Can you work these out from the model? Positions are in its coordinate system, mm. A direction names the side the tool comes from. Round coordinates to 2 decimals unless told otherwise and drop trailing zeros. Write each loop counter-clockwise with the first axis right and the second up, starting at its lowest first coordinate (ties: lowest second). Pieces come first, ordered by that corner, then holes. Notation, with made-up numbers: (-19.75, 58.25) - (-10.75, 58.25) arc R7 ccw to (-10.75, 70.25) - close; hole circle Ø7 at (56, 66.5). An arc over 180 degrees is marked (long way). One line per item, written item: value. Start each with the question number.
(1) On a 3-axis mill with a long thin cutter (end or side, diameter ignored), from which of +Z, -Z, +X, -X, +Y, -Y can I reach the whole of each face in a straight line? I mean faces 4 (the face through (6, 101, 12.7)), 5 (the face through (-10, 99, 15)). Say none if no direction works.
(2) I want a section at B-B on z = 0. List the corners of the cut face in (x, y) for me.
(3) Thinking about a two-plate mould opening in Z: for faces 1 (the face through (-7.83, 101.4, -6.38)), 2 (the face through (9, 99, -15)), 3 (the face through (15, 99, 10)), which applies, +Z half, -Z half, draft (parallel to the pull), parting line (faces both ways), or undercut?
(4) I'm going to push flat-ended pins straight in: pin 1 Ø4.5 at (y, z) = (75, 0.5) entering from +X; pin 2 Ø4.5 at (x, y) = (-0.5, 116) entering from -Z. Where does each tip first touch, or does it pass through?
(5) I want a section at A-A on x = 0. List the corners of the cut face in (y, z) for me, plus the area to 3 significant figures.
(6) If I drill on L1, parallel to X at y = 55, z = -11.75; L2, parallel to Z at x = 4.5, y = 11.5, over which ranges is the centre line in solid material (lowest first)? Write a range as from..to.
from build123d import *

# Parameters (mm, degrees)
CROQUIS1_W              = 30
CROQUIS1_H              = 30
SALIENTE_EXTRUIR1_DEPTH = 200
CROQUIS3_R              = 3.5
CORTAR_EXTRUIR2_DEPTH   = 202.121853611


with BuildPart() as part:
    # Croquis1 → Saliente-Extruir1 (new body)
    with BuildSketch(Plane(origin=(0, 0, 0), x_dir=(1, 0, 0), z_dir=(0, 1, 0))):
        Rectangle(CROQUIS1_W, CROQUIS1_H)
    extrude(amount=SALIENTE_EXTRUIR1_DEPTH)

    # Croquis3 → Cortar-Extruir2 (cut, through all)
    with BuildSketch(Plane(origin=(0, 200, 0), x_dir=(1, 0, 0), z_dir=(0, 1, 0))):
        with Locations(Location((0, 0, 0), (0, 0, 270))):
            Circle(CROQUIS3_R)
        with BuildLine():
            Line((4, 15), (-4, 15))
            Line((-4, 15), (-4, 13.2))
            ThreePointArc((-4, 13.2), (-4.146446609, 12.846446609), (-4.5, 12.7))
            Line((-4.5, 12.7), (-7.75, 12.7))
            ThreePointArc((-7.75, 12.7), (-8.103553391, 12.553553391), (-8.25, 12.2))
            Line((-8.25, 12.2), (-8.25, 9.907106781))
            ThreePointArc((-8.25, 9.907106781), (-8.211939766, 9.715765065), (-8.103553391, 9.553553391))
            Line((-8.103553391, 9.553553391), (-4.696446609, 6.146446609))
            ThreePointArc((-4.696446609, 6.146446609), (-4.534234935, 6.038060234), (-4.342893219, 6))
            Line((-4.342893219, 6), (4.342893219, 6))
            ThreePointArc((4.342893219, 6), (4.534234935, 6.038060234), (4.696446609, 6.146446609))
            Line((4.696446609, 6.146446609), (8.103553391, 9.553553391))
            ThreePointArc((8.103553391, 9.553553391), (8.211939766, 9.715765065), (8.25, 9.907106781))
            Line((8.25, 9.907106781), (8.25, 12.2))
            ThreePointArc((8.25, 12.2), (8.103553391, 12.553553391), (7.75, 12.7))
            Line((7.75, 12.7), (4.5, 12.7))
            ThreePointArc((4.5, 12.7), (4.146446609, 12.846446609), (4, 13.2))
            Line((4, 13.2), (4, 15))
        make_face()
        with BuildLine():
            Line((6, 4.342893219), (6, -4.342893219))
            ThreePointArc((6, -4.342893219), (6.038060234, -4.534234935), (6.146446609, -4.696446609))
            Line((6.146446609, -4.696446609), (9.553553391, -8.103553391))
            ThreePointArc((9.553553391, -8.103553391), (9.715765065, -8.211939766), (9.907106781, -8.25))
            Line((9.907106781, -8.25), (12.2, -8.25))
            ThreePointArc((12.2, -8.25), (12.553553391, -8.103553391), (12.7, -7.75))
            Line((12.7, -7.75), (12.7, -4.5))
            ThreePointArc((12.7, -4.5), (12.846446609, -4.146446609), (13.2, -4))
            Line((13.2, -4), (15, -4))
            Line((15, -4), (15, 4))
            Line((15, 4), (13.2, 4))
            ThreePointArc((13.2, 4), (12.846446609, 4.146446609), (12.7, 4.5))
            Line((12.7, 4.5), (12.7, 7.75))
            ThreePointArc((12.7, 7.75), (12.553553391, 8.103553391), (12.2, 8.25))
            Line((12.2, 8.25), (9.907106781, 8.25))
            ThreePointArc((9.907106781, 8.25), (9.715765065, 8.211939766), (9.553553391, 8.103553391))
            Line((9.553553391, 8.103553391), (6.146446609, 4.696446609))
            ThreePointArc((6.146446609, 4.696446609), (6.038060234, 4.534234935), (6, 4.342893219))
        make_face()
        with BuildLine():
            Line((4.342893219, -6), (-4.342893219, -6))
            ThreePointArc((-4.342893219, -6), (-4.534234935, -6.038060234), (-4.696446609, -6.146446609))
            Line((-4.696446609, -6.146446609), (-8.103553391, -9.553553391))
            ThreePointArc((-8.103553391, -9.553553391), (-8.211939766, -9.715765065), (-8.25, -9.907106781))
            Line((-8.25, -9.907106781), (-8.25, -12.2))
            ThreePointArc((-8.25, -12.2), (-8.103553391, -12.553553391), (-7.75, -12.7))
            Line((-7.75, -12.7), (-4.5, -12.7))
            ThreePointArc((-4.5, -12.7), (-4.146446609, -12.846446609), (-4, -13.2))
            Line((-4, -13.2), (-4, -15))
            Line((-4, -15), (4, -15))
            Line((4, -15), (4, -13.2))
            ThreePointArc((4, -13.2), (4.146446609, -12.846446609), (4.5, -12.7))
            Line((4.5, -12.7), (7.75, -12.7))
            ThreePointArc((7.75, -12.7), (8.103553391, -12.553553391), (8.25, -12.2))
            Line((8.25, -12.2), (8.25, -9.907106781))
            ThreePointArc((8.25, -9.907106781), (8.211939766, -9.715765065), (8.103553391, -9.553553391))
            Line((8.103553391, -9.553553391), (4.696446609, -6.146446609))
            ThreePointArc((4.696446609, -6.146446609), (4.534234935, -6.038060234), (4.342893219, -6))
        make_face()
        with BuildLine():
            Line((-6, -4.342893219), (-6, 4.342893219))
            ThreePointArc((-6, 4.342893219), (-6.038060234, 4.534234935), (-6.146446609, 4.696446609))
            Line((-6.146446609, 4.696446609), (-9.553553391, 8.103553391))
            ThreePointArc((-9.553553391, 8.103553391), (-9.715765065, 8.211939766), (-9.907106781, 8.25))
            Line((-9.907106781, 8.25), (-12.2, 8.25))
            ThreePointArc((-12.2, 8.25), (-12.553553391, 8.103553391), (-12.7, 7.75))
            Line((-12.7, 7.75), (-12.7, 4.5))
            ThreePointArc((-12.7, 4.5), (-12.846446609, 4.146446609), (-13.2, 4))
            Line((-13.2, 4), (-15, 4))
            Line((-15, 4), (-15, -4))
            Line((-15, -4), (-13.2, -4))
            ThreePointArc((-13.2, -4), (-12.846446609, -4.146446609), (-12.7, -4.5))
            Line((-12.7, -4.5), (-12.7, -7.75))
            ThreePointArc((-12.7, -7.75), (-12.553553391, -8.103553391), (-12.2, -8.25))
            Line((-12.2, -8.25), (-9.907106781, -8.25))
            ThreePointArc((-9.907106781, -8.25), (-9.715765065, -8.211939766), (-9.553553391, -8.103553391))
            Line((-9.553553391, -8.103553391), (-6.146446609, -4.696446609))
            ThreePointArc((-6.146446609, -4.696446609), (-6.038060234, -4.534234935), (-6, -4.342893219))
        make_face()
    extrude(amount=-CORTAR_EXTRUIR2_DEPTH, mode=Mode.SUBTRACT)


solid = part.part
Established:
1. face 4: +Y, -Y
1. face 5: +Z, +X, -X, +Y, -Y
2. outline: (-6, 0) - (-3.5, 0) - (-3.5, 200) - (-6, 200) - close; (3.5, 0) - (6, 0) - (6, 200) - (3.5, 200) - close
3. face 1: undercut
3. face 2: -Z half
3. face 3: draft
4. pin 1: x = 6
4. pin 2: z = -6
5. outline: (0, -6) - (200, -6) - (200, -3.5) - (0, -3.5) - close; (0, 3.5) - (200, 3.5) - (200, 6) - (0, 6) - close
5. area: 1,000 mm2
6. L1: -15..-8.25, 8.25..15
6. L2: -15..-12.7, -6.03..6.03, 12.7..15
